Work out the finished part from the listing and answer in its coordinate system (mm). A direction names the side the tool comes from. Give positions to 0.01 mm unless a question says otherwise; leave off trailing zeros. Loops run counter-clockwise (first coordinate to the right, second up) from the corner with the lowest first, then second, coordinate; pieces in that order, holes last. Notation, with made-up numbers: (23, 82) - (57, 82) arc R16 ccw to (57, 113) - close; hole circle Ø8 at (2, 60). An arc over 180 degrees is marked (long way). Use one line per item in the form item = value. Start each with the question number.
from build123d import *

# Parameters (mm, degrees)
SKETCH2_R          = 1.5
CUT_EXTRUDE1_DEPTH = 5


with BuildPart() as part:
    # Sketch1 → Revolve1 (revolve)
    with BuildSketch(Plane(origin=(0, 0, 0), x_dir=(1, 0, 0), z_dir=(0, 1, 0))):
        Polygon((0, 0), (11, 0), (11, 3.06822983), (3.73856208, 3.06822983), (3.73856208, 6.631290685), (13.75, 6.631290685), (13.75, 16.896299341), (7.819804578, 19.35), (2.5, 19.35), (2.5, 31.35), (0, 31.35), align=None)
    revolve(axis=Axis((0, 0, -31.35), (0, 0, 1)))

    # Sketch2 → Cut-Extrude1 (cut)
    with BuildSketch(Plane.XY):
        with Locations((8.298889382, 0)):
            Circle(SKETCH2_R)
        with Locations((0, -8.298889382)):
            Circle(SKETCH2_R)
        with Locations((-8.298889382, 0)):
            Circle(SKETCH2_R)
        with Locations((0, 8.298889382)):
            Circle(SKETCH2_R)
    extrude(amount=-CUT_EXTRUDE1_DEPTH, mode=Mode.SUBTRACT)


solid = part.part
1) Determine the mould class of faces 5 (the flat face through (-3, -3, -6.631)), 6 (the cylindrical face through (0.81, 9.56, -1.51)), 7 (the flat face through (-2, 2, -19.35)) for opening direction Z: released by +Z, released by -Z, zero draft, split by the parting line, or undercut.
2) A cutting plane is placed at C-C (z = -10). Give the vertices of the cut face in (x, y).
3) A tool of negligible diameter and unlimited length cuts with its end or side. For faces 1 (the flat face through (0, 0, 0)), 2 (the cylindrical face through (-6.91, -0.57, -1.51)), 3 (the cylindrical face through (3.453, -1.432, -4.875)), 4 (the cylindrical face through (-0.54, -2.44, -25.43)), from which of +Z, -Z, +X, -X, +Y, -Y can it reach the whole face along a straight path? Write none if from no direction.
4) Find the intervals of material crossed by probe 1 along Y at (x, z) = (0, -1.7); probe 2 along Z at (x, y) = (-2.5, 4.75); probe 3 along Z at (x, y) = (-2.75, 1.75), in increasing order.
5) A cutting plane is placed at D-D (z = -26). Give the vertices of the cut face in (x, y), plus the area to 3 significant figures.
6) Flat-ended cylindrical pins translate along their axes: pin 1 Ø1.5 at (x, z) = (-4.5, -15) entering from -Y; pin 2 Ø2.5 at (x, y) = (-8.3, 0) entering from +Z; pin 3 Ø1 at (x, z) = (-6.5, -9.5) entering from -Y. Find the tip coordinate at first contact, or state that the pin passes through.
7) A cutting plane is placed at A-A (x = 0). Give the vertices of the cut face in (y, z), plus the area to 3 significant figures.
Answer sheet:
q1.face_5 = undercut
q1.face_6 = zero draft
q1.face_7 = released by -Z
q2.outline = circle Ø27.5 at (0, 0)
q3.face_1 = +Z, +X, -X, +Y, -Y
q3.face_2 = +Z
q3.face_3 = none
q3.face_4 = -Z
q4.probe_1 = -11 to -9.8, -6.8 to 6.8, 9.8 to 11
q4.probe_2 = -19.35 to -6.63, -3.07 to 0
q4.probe_3 = -19.35 to 0
q5.outline = circle Ø5 at (0, 0)
q5.area = 19.6 mm²
q6.pin_1 = -13.23
q6.pin_2 = -6.63
q6.pin_3 = -12.37
q7.outline = (-13.75, -16.9) - (-7.82, -19.35) - (-2.5, -19.35) - (-2.5, -31.35) - (2.5, -31.35) - (2.5, -19.35) - (7.82, -19.35) - (13.75, -16.9) - (13.75, -6.63) - (3.74, -6.63) - (3.74, -3.07) - (6.8, -3.07) - (6.8, 0) - (-6.8, 0) - (-6.8, -3.07) - (-3.74, -3.07) - (-3.74, -6.63) - (-13.75, -6.63) - close; (-11, -3.07) - (-9.8, -3.07) - (-9.8, 0) - (-11, 0) - close; (9.8, -3.07) - (11, -3.07) - (11, 0) - (9.8, 0) - close
q7.area = 471 mm²
